Could you check a few things on this drawing? It's one solid part, dimensions in mm from its lowest x, y, z. A direction names the side the tool comes from. Give positions to 0.01 mm unless a question says otherwise; leave off trailing zeros. Order: outer loops, then holes, each group sorted by start corner. A loop starts at its lowest first (then second) coordinate and runs counter-clockwise, first axis right, second up. Notation, with made-up numbers: (13.25, 53) - (60.25, 53) arc R14 cw to (60.25, 71) - close; hole circle Ø4 at (85, 69). An arc over 180 degrees is marked (long way). Answer as CSV lines item,"result".
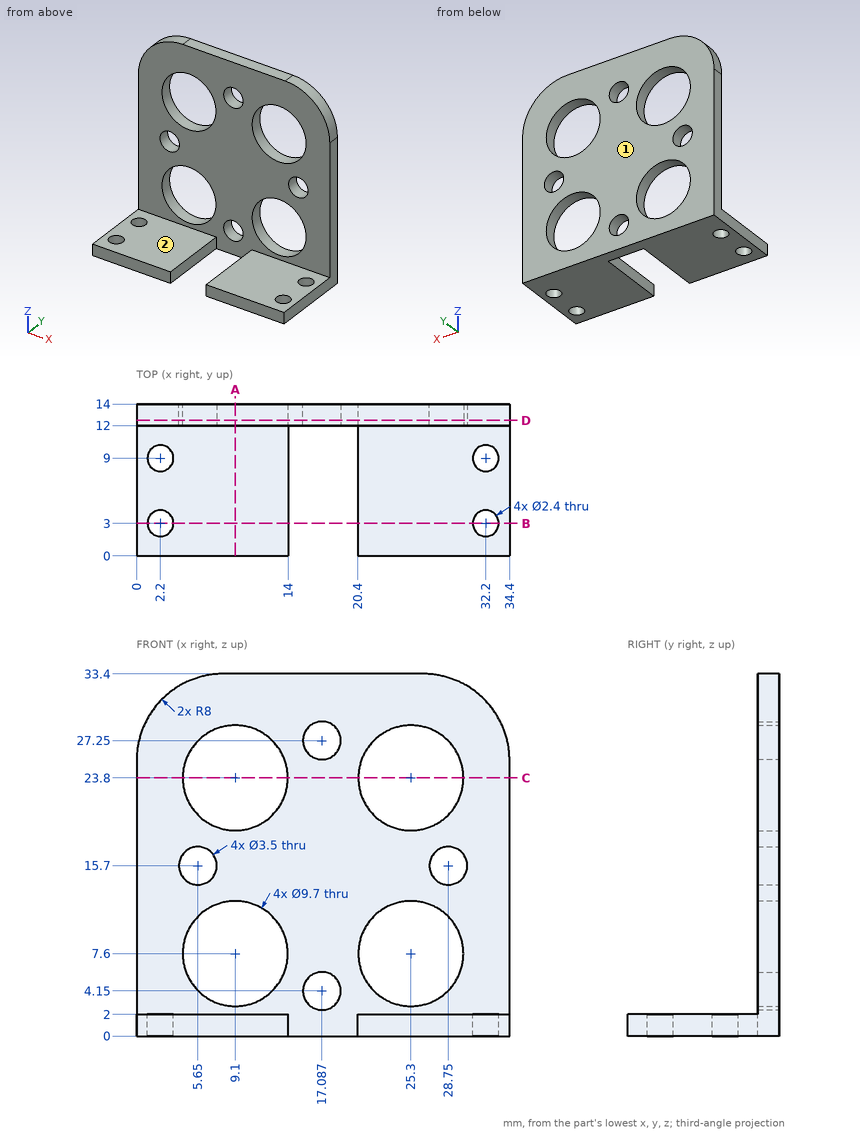
1) I need wall thicknesses on line 1 along Z through (x, y) = (9.1, 12.95); line 2 along Y through (x, z) = (2.2, 1.25); line 3 along Y through (x, z) = (16, 6.5). Which ranges of each line are inside material? Lowest first, please. Write a range as [from, to].
Answer block:
line 1,"[0, 2.75], [12.45, 18.95], [28.65, 33.4]"
line 2,"[0, 1.8], [4.2, 7.8], [10.2, 14]"
line 3,"[12, 14]"
2) I want a section at C-C on z = 23.8. Write out the boundary of the cut face in (x, y), plus the area to 3 significant figures.
Answer block:
outline,"(0, 12) - (4.25, 12) - (4.25, 14) - (0, 14) - close; (13.95, 12) - (20.45, 12) - (20.45, 14) - (13.95, 14) - close; (30.15, 12) - (34.4, 12) - (34.4, 14) - (30.15, 14) - close"
area,"30.0 mm2"
3) I want a section at A-A on x = 9.1. Write out the boundary of the cut face in (y, z).
Answer block:
outline,"(0, 0) - (14, 0) - (14, 2.75) - (12, 2.75) - (12, 2) - (0, 2) - close; (12, 12.45) - (14, 12.45) - (14, 18.95) - (12, 18.95) - close; (12, 28.65) - (14, 28.65) - (14, 33.4) - (12, 33.4) - close"
4) I want a section at D-D on y = 12.5. Count the separate pieces of the cut face and the enclosed holes in it, plus the area to 3 significant figures.
Answer block:
separate pieces,"1"
enclosed holes,"8"
area,"787 mm2"
5) I want a section at B-B on y = 3. Write out the boundary of the cut face in (x, z), plus the area to 3 significant figures.
Answer block:
outline,"(0, 0) - (1, 0) - (1, 2) - (0, 2) - close; (3.4, 0) - (14, 0) - (14, 2) - (3.4, 2) - close; (20.4, 0) - (31, 0) - (31, 2) - (20.4, 2) - close; (33.4, 0) - (34.4, 0) - (34.4, 2) - (33.4, 2) - close"
area,"46.4 mm2"
6) Which directions (+Z, -Z, +X, -X, +Y, -Y) give clear straight access to the entire face, cutting with the end or side of a thin tool? Please do the marked faces 1 and 2.
Answer block:
face 1,"+Z, -Z, +X, -X, +Y"
face 2,"+Z, +X, -X, -Y"
7) I'm going to push flat-ended pins straight in: P1, Ø4, axis at x = 2.2, y = 3, coming from the +Z side; P2, Ø4.5, axis at x = 28.75, z = 15.7, coming from the +Y side; P3, Ø2, axis at x = 5.65, z = 15.7, coming from the +Y side; P4, Ø3, axis at x = 9, z = 18, coming from the -Y side. Where does each tip first touch, or does it pass through?
Answer block:
P1,"z = 2"
P2,"y = 14"
P3,"through"
P4,"y = 12"
